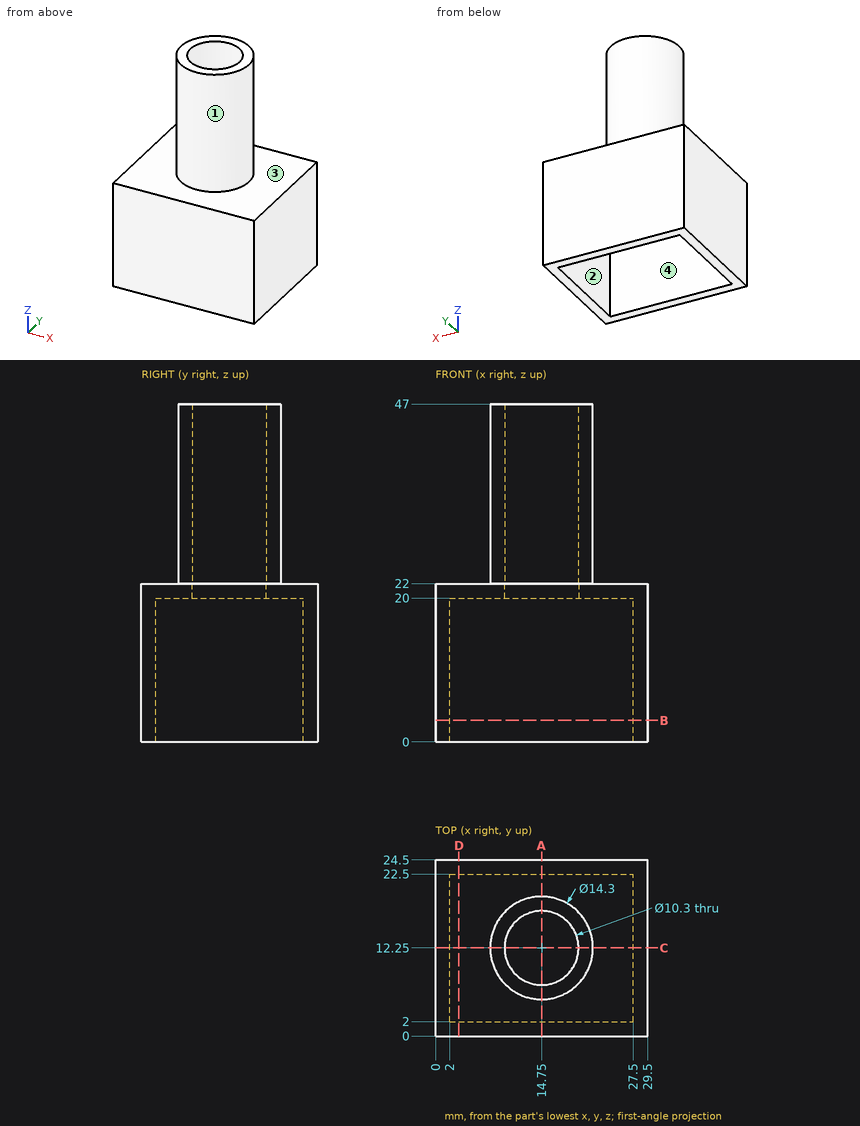
Verification items for this drawing (mm, ordinates from the low corner). Give positions to 0.01 mm unless a question says otherwise; leave off trailing zeros. Write each loop counter-clockwise with the first axis right and the second up, starting at its lowest first coordinate (ties: lowest second). Pieces come first, ordered by that corner, then holes. Notation, with made-up numbers: (6.25, 55) - (50.25, 55) arc R15 ccw to (50.25, 66) - close; hole circle Ø11 at (-13, -33). An arc over 180 degrees is marked (long way). Answer as a JSON object with one key per item and string values. Group by question number.
1) Depth check by flat-ended pin: P1, Ø4, axis at x = 13, y = 13.5, coming from the -Z side; P2, Ø8, axis at x = 8.5, y = 7, coming from the +Z side; P3, Ø4, axis at x = 14, z = 32.5, coming from the -Y side; P4, Ø4, axis at y = 6.5, z = 35.5, coming from the -X side. Enter the tip coordinate at first touch or a pass-through.
2) Sectioned sample at A-A (x = 14.75). Record the cut outline in (y, z), then the cut area to 3 significant figures.
3) Sectioned sample at B-B (z = 3). Record the cut outline in (x, y), then the cut area to 3 significant figures.
4) Thickness scan on probe 1 along X at (y, z) = (13.5, 6.5); probe 2 along Y at (x, z) = (14.75, 32.5); probe 3 along Y at (x, z) = (14.75, 21.3). Record the ranges inside material, lowest first. Write a range as from..to.
5) Release check for a two-part mould opening along Y. For the marked faces 1, 2, 3 and 4 record: pulls with the +Y half, pulls with the -Y half, needs draft (parallel to the pull), parting line crosses it, or undercut.
6) Sectioned sample at D-D (x = 3.25). Record the cut outline in (y, z).
7) Sectioned sample at C-C (y = 12.25). Record the cut outline in (x, z), then the cut area to 3 significant figures.
Geometry results:
{
 "1": {"P1": "passes through", "P2": "stops at z = 47", "P3": "stops at y = 5.1", "P4": "stops at x = 8.66"},
 "2": {"outline": "(0, 0) - (2, 0) - (2, 20) - (7.1, 20) - (7.1, 47) - (5.1, 47) - (5.1, 22) - (0, 22) - close; (17.4, 20) - (22.5, 20) - (22.5, 0) - (24.5, 0) - (24.5, 22) - (19.4, 22) - (19.4, 47) - (17.4, 47) - close", "area": "208 mm^2"},
 "3": {"outline": "(0, 0) - (29.5, 0) - (29.5, 24.5) - (0, 24.5) - close; hole (2, 2) - (27.5, 2) - (27.5, 22.5) - (2, 22.5) - close", "area": "200 mm^2"},
 "4": {"probe 1": "x = 0..2, 27.5..29.5", "probe 2": "y = 5.1..7.1, 17.4..19.4", "probe 3": "y = 0..7.1, 17.4..24.5"},
 "5": {"face 1": "parting line crosses it", "face 2": "undercut", "face 3": "needs draft", "face 4": "undercut"},
 "6": {"outline": "(0, 0) - (2, 0) - (2, 20) - (22.5, 20) - (22.5, 0) - (24.5, 0) - (24.5, 22) - (0, 22) - close"},
 "7": {"outline": "(0, 0) - (2, 0) - (2, 20) - (9.6, 20) - (9.6, 47) - (7.6, 47) - (7.6, 22) - (0, 22) - close; (19.9, 20) - (27.5, 20) - (27.5, 0) - (29.5, 0) - (29.5, 22) - (21.9, 22) - (21.9, 47) - (19.9, 47) - close", "area": "218 mm^2"}
}
